from build123d import *

# Parameters (mm, degrees)
SKETCH1_W                       = 90
SKETCH1_H                       = 15
BOSS_EXTRUDE1_DEPTH             = 60
SKETCH3_R                       = 30
SKETCH3_R_2                     = 25
SKETCH4_R                       = 55
SKETCH4_R_2                     = 25
BOSS_EXTRUDE2_DEPTH             = 12
M8X1_0_TAPPED_HOLE1_D           = 7
M8X1_0_TAPPED_HOLE1_CSINK_D     = 8.05
M8X1_0_TAPPED_HOLE1_CSINK_ANGLE = 90
FILLET1_R                       = 7.5
HOLE2_D                         = 10
HOLE2_CBORE_D                   = 18
HOLE2_CBORE_DEPTH               = 6
MIRROR2_COPY_1_D                = 10
MIRROR2_COPY_1_CBORE_D          = 18
MIRROR2_COPY_1_CBORE_DEPTH      = 6
HOLE3_D                         = 5
BOSS_EXTRUDE3_REACH             = 239.363
HOLE4_REACH                     = 239.363
HOLE4_BORE_R                    = 12.5


# Read off the part's stored shape, not the designer's step: CirPattern1
with BuildPart() as part:
    # Sketch1 → Boss-Extrude1 (new, symmetric)
    with BuildSketch(Plane.XY):
        Rectangle(SKETCH1_W, SKETCH1_H)
    extrude(amount=BOSS_EXTRUDE1_DEPTH, both=True)

    # Sweep1: sweep along a path in Sketch2
    with BuildLine(Plane.XY) as sweep1_path:
        Line((0, 7.5), (0, 12.5))
        ThreePointArc((0, 12.5), (16.076951546, 72.5), (60, 116.423048454))
        Line((60, 116.423048454), (77.320508076, 126.423048454))
    # Sketch3 → Sweep1 (sweep)
    with BuildSketch(Plane(origin=(0, 7.5, 0), x_dir=(1, 0, 0), z_dir=(0, 1, 0))):
        Circle(SKETCH3_R)
        Circle(SKETCH3_R_2, mode=Mode.SUBTRACT)
    sweep(path=sweep1_path.line)

    # Sketch4 → Boss-Extrude2 (add)
    with BuildSketch(Plane(origin=(112.733166849, 65.086524227, 0), x_dir=(0, 0, -1), z_dir=(0.8660254037844357, 0.5000000000000052, 0))):
        with Locations(Location((0, 70.825317547, 0), (0, 0, 90))):
            Circle(SKETCH4_R)
        with Locations(Location((0, 70.825317547, 0), (0, 0, 90))):
            Circle(SKETCH4_R_2, mode=Mode.SUBTRACT)
    extrude(amount=-BOSS_EXTRUDE2_DEPTH)

    # M8x1.0 Tapped Hole1 (through all)
    with Locations(Plane(origin=(112.733166849, 65.086524227, 0), x_dir=(0, 0, -1), z_dir=(0.8660254037844357, 0.5000000000000052, 0))):
        with Locations((45, 70.825317547)):
            CounterSinkHole(M8X1_0_TAPPED_HOLE1_D / 2, M8X1_0_TAPPED_HOLE1_CSINK_D / 2, counter_sink_angle=M8X1_0_TAPPED_HOLE1_CSINK_ANGLE)

    # CirPattern1 outline → CirPattern1 (revolve, cut)
    with BuildSketch(Plane(origin=(-15.927087189, 27.586524227, -22.5), x_dir=(0.5000000000000049, -0.8660254037844358, 0), z_dir=(0, 0, 1))):
        Polygon((0, 118.173048454), (3.5, 118.173048454), (3.5, 129.648048454), (4.025, 130.173048454), (0, 130.173048454), align=None)
    revolve(axis=Axis((-15.927087189, 27.586524227, -22.5), (0.8660254037844358, 0.5000000000000049, 0)), mode=Mode.SUBTRACT)

    # CirPattern1 2 outline → CirPattern1 2 (revolve, cut)
    with BuildSketch(Plane(origin=(-15.927087189, 27.586524227, 22.5), x_dir=(0.500000000000004, -0.8660254037844363, 0), z_dir=(0, 0, 1))):
        Polygon((0, 118.173048454), (3.5, 118.173048454), (3.5, 129.648048454), (4.025, 130.173048454), (0, 130.173048454), align=None)
    revolve(axis=Axis((-15.927087189, 27.586524227, 22.5), (0.8660254037844363, 0.500000000000004, 0)), mode=Mode.SUBTRACT)

    # CirPattern1 3 outline → CirPattern1 3 (revolve, cut)
    with BuildSketch(Plane(origin=(-35.412658774, 61.336524227, 45), x_dir=(0.500000000000004, -0.8660254037844363, 0), z_dir=(0, 0, 1))):
        Polygon((0, 118.173048454), (3.5, 118.173048454), (3.5, 129.648048454), (4.025, 130.173048454), (0, 130.173048454), align=None)
    revolve(axis=Axis((-35.412658774, 61.336524227, 45), (0.8660254037844363, 0.500000000000004, 0)), mode=Mode.SUBTRACT)

    # CirPattern1 4 outline → CirPattern1 4 (revolve, cut)
    with BuildSketch(Plane(origin=(-54.898230359, 95.086524227, 22.5), x_dir=(0.5000000000000049, -0.8660254037844358, 0), z_dir=(0, 0, 1))):
        Polygon((0, 118.173048454), (3.5, 118.173048454), (3.5, 129.648048454), (4.025, 130.173048454), (0, 130.173048454), align=None)
    revolve(axis=Axis((-54.898230359, 95.086524227, 22.5), (0.8660254037844358, 0.5000000000000049, 0)), mode=Mode.SUBTRACT)

    # CirPattern1 5 outline → CirPattern1 5 (revolve, cut)
    with BuildSketch(Plane(origin=(-54.898230359, 95.086524227, -22.5), x_dir=(0.5000000000000049, -0.8660254037844358, 0), z_dir=(0, 0, 1))):
        Polygon((0, 118.173048454), (3.5, 118.173048454), (3.5, 129.648048454), (4.025, 130.173048454), (0, 130.173048454), align=None)
    revolve(axis=Axis((-54.898230359, 95.086524227, -22.5), (0.8660254037844358, 0.5000000000000049, 0)), mode=Mode.SUBTRACT)

    # Fillet1
    fillet1_edges = [part.edges().sort_by_distance(p)[0] for p in [
        (-45, 0, 60),
        (45, 0, 60),
        (-45, 0, -60),
        (45, 0, -60),
    ]]
    fillet(fillet1_edges, radius=FILLET1_R)

    # Hole2 (through all)
    with Locations(Plane(origin=(0, 7.5, 0), x_dir=(1, 0, 0), z_dir=(0, 1, 0))):
        with Locations((-30, 45)):
            hole2 = CounterBoreHole(HOLE2_D / 2, HOLE2_CBORE_D / 2, HOLE2_CBORE_DEPTH)

    # Mirror1: Hole2 across plane
    add(hole2.mirror(Plane(origin=(0, 0, 0), x_dir=(0, 0, 1), z_dir=(1, 0, 0))), mode=Mode.SUBTRACT)

    # Mirror2: Hole2 across plane
    add(hole2.mirror(Plane.XY), mode=Mode.SUBTRACT)

    # Mirror2 copy 1 (through all)
    with Locations(Plane(origin=(0, 7.5, 0), x_dir=(-1, 0, 0), z_dir=(0, 1, 0))):
        with Locations((-30, 45)):
            CounterBoreHole(MIRROR2_COPY_1_D / 2, MIRROR2_COPY_1_CBORE_D / 2, MIRROR2_COPY_1_CBORE_DEPTH)

    # Hole3 (through all)
    with Locations(Plane(origin=(0, 7.5, 0), x_dir=(1, 0, 0), z_dir=(0, 1, 0))):
        with Locations((0, 45)):
            hole3 = Hole(HOLE3_D / 2)

    # Mirror3: Hole3 across plane
    add(hole3.mirror(Plane.XY), mode=Mode.SUBTRACT)

    # Sketch14 → Boss-Extrude3 (add, up to next)
    with BuildSketch(Plane(origin=(-45, 0, 0), x_dir=(0, 0, -1), z_dir=(1, 0, 0)), mode=Mode.PRIVATE) as boss_extrude3_sk1:
        with BuildLine():
            Line((6, 30.921215972), (6, -7.5))
            Line((6, -7.5), (-6, -7.5))
            Line((-6, -7.5), (-6, 30.921215972))
            ThreePointArc((-6, 30.921215972), (0, 70), (6, 30.921215972))
        make_face()
    boss_extrude3_tool1 = extrude(boss_extrude3_sk1.sketch, amount=BOSS_EXTRUDE3_REACH, mode=Mode.PRIVATE) - part.part
    add(boss_extrude3_tool1.solids().sort_by_distance((-45, 39.762246, 0))[0])

    # Hole4 bore → Hole4 (cut, up to next)
    with BuildSketch(Plane.ZY.offset(45), mode=Mode.PRIVATE) as hole4_sk1:
        with Locations((0, 50)):
            Circle(HOLE4_BORE_R)
    hole4_tool1 = extrude(hole4_sk1.sketch, amount=-HOLE4_REACH, mode=Mode.PRIVATE) & part.part
    add(hole4_tool1.solids().sort_by_distance((-45, 50, 0))[0], mode=Mode.SUBTRACT)


solid = part.part
Model file for the job. Use its own axes, mm. A direction names the side the tool comes from. Give positions to 0.01 mm unless a question says otherwise; leave off trailing zeros. Write each loop counter-clockwise with the first axis right and the second up, starting at its lowest first coordinate (ties: lowest second). Pieces come first, ordered by that corner, then holes. Notation, with made-up numbers: (48.5, 81) - (88.5, 81) arc R17 cw to (88.5, 105) - close; hole circle Ø2 at (70, 13.5). An arc over 180 degrees is marked (long way). Answer as CSV lines item,"result".
1. Two-plate mould, pull along X, no slides. Class faces 1 (the face through (-26, 1.5, 41)), 2 (the face through (-1, 0, -60)), 3 (the face through (-36.633, 4.542, -51.083)), 4 (the face through (45, 0, 1)): +X half, -X half, draft (parallel to the pull), parting line (faces both ways), or undercut.
Responses:
face 1,"undercut"
face 2,"draft"
face 3,"undercut"
face 4,"+X half"
2. Band-saw the part on B-B (x = 0). Count the separate pieces of the cut face and the enclosed holes in it, and give its area (3 significant figures).
Responses:
separate pieces,"3"
enclosed holes,"1"
area,"2,850 mm2"
3. Band-saw the part on A-A (z = 0). Write the cut outline in (x, y), and give its area (3 significant figures).
Responses:
outline,"(-45, -7.5) - (45, -7.5) - (45, 7.5) - (30, 7.5) - (30, 12.5) arc R90 cw to (75, 90.44) - (81.93, 94.44) - (94.43, 72.79) - (104.82, 78.79) - (89.82, 104.77) - (72.5, 94.77) arc R95 ccw to (25, 12.5) - (25, 7.5) - (-25, 7.5) - (-25, 12.5) arc R145 cw to (-22.83, 37.5) - (-45, 37.5) - close; (-45, 62.5) - (-16.11, 62.5) arc R145 cw to (47.5, 138.07) - (64.82, 148.07) - (49.82, 174.05) - (39.43, 168.05) - (51.93, 146.4) - (45, 142.4) arc R150 ccw to (-18.54, 70) - (-45, 70) - close"
area,"3,980 mm2"
4. 3-axis set-ups, long thin cutter, end or side, ignore diameter. For faces 5 (the face through (-30.875, 69.984, 0.794)), 6 (the face through (55.09, 140.93, -23.67)), 7 (the face through (-31.172, 4.542, 53.923)): which of +Z, -Z, +X, -X, +Y, -Y reach the whole face in a straight line?
Responses:
face 5,"-X"
face 6,"none"
face 7,"+Y"
5. Drill centre lines: L1, parallel to Z at x = -30, y = -2; L2, parallel to X at y = -3, z = -45; L3, parallel to Z at x = 30, y = 4. Where is each one in solid material? Low to high. Write a range as [from, to].
Responses:
L1,"z = [-60, -50], [-40, 40], [50, 60]"
L2,"x = [-45, -35], [-25, -2.5], [2.5, 25], [35, 45]"
L3,"z = [-60, -54], [-36, 36], [54, 60]"
6. Pin check, flat tips, straight feed: pin 1 (12 mm diameter, centred on x = 11.5, y = 33, fed in from +Z); pin 2 (14.5 mm diameter, centred on x = 30, z = 48, fed in from +Y); pin 3 (11 mm diameter, centred on x = -30, z = -45, fed in from +Y). Stop position of each tip, or through.
Responses:
pin 1,"stops at z = 29.79"
pin 2,"stops at y = 7.5"
pin 3,"stops at y = 1.5"
